```python
from build123d import *

# Parameters (mm, degrees)
SKETCH1_R           = 6
SKETCH1_R_2         = 3.5
BOSS_EXTRUDE1_DEPTH = 2
SKETCH2_R           = 4.5
BOSS_EXTRUDE2_DEPTH = 3
SKETCH3_R           = 2.5
CUT_EXTRUDE1_DEPTH  = 35.398401126
CUT_EXTRUDE2_DEPTH  = 35.398401126


with BuildPart() as part:
    # Sketch1 → Boss-Extrude1 (new body)
    with BuildSketch(Plane.XY):
        Circle(SKETCH1_R)
        with Locations((30, 0)):
            Circle(SKETCH1_R_2)
        Polygon((30, 3.5), (0, 6), (0, -6), (30, -3.5), align=None)
    extrude(amount=BOSS_EXTRUDE1_DEPTH)

    # Sketch2 → Boss-Extrude2 (add)
    with BuildSketch(Plane.XY.offset(2)):
        Circle(SKETCH2_R)
    extrude(amount=BOSS_EXTRUDE2_DEPTH)

    # Sketch3 → Cut-Extrude1 (cut, through all)
    with BuildSketch(Plane.XY.offset(5)):
        Circle(SKETCH3_R)
    extrude(amount=-CUT_EXTRUDE1_DEPTH, mode=Mode.SUBTRACT)

    # Sketch4 → Cut-Extrude2 (cut, through all)
    with BuildSketch(Plane(origin=(0, 0, 0), x_dir=(-1, 0, 0), z_dir=(0, 0, -1))):
        with BuildLine():
            ThreePointArc((-29, 0), (-29.292893219, 0.707106781), (-30, 1))
            Line((-30, 1), (-30, -1))
            ThreePointArc((-30, -1), (-29.292893219, -0.707106781), (-29, 0))
        make_face()
        with BuildLine():
            Line((-30, -1), (-30, 1))
            ThreePointArc((-30, 1), (-31, 0), (-30, -1))
        make_face()
    extrude(amount=-CUT_EXTRUDE2_DEPTH, mode=Mode.SUBTRACT)


solid = part.part
```
Read the model definition and answer for the solid it produces. Units are mm, in the model's axes. Coordinates: 2 decimals unless noted, no trailing zeros. Order: outer loops, then holes, each group sorted by start corner. A loop starts at its lowest first (then second) coordinate and runs counter-clockwise, first axis right, second up. Notation, with made-up numbers: (87.5, 82.25) - (109.5, 82.25) arc R25 ccw to (109.5, 98.25) - close; hole circle Ø7 at (-20, 22.25). An arc over 180 degrees is marked (long way). Answer as a JSON object with one key per item and string values. Group by question number.
Item 1: Section B-B (z = 1.15) is taken. Give the vertices of the cut face in (x, y), plus the area to 3 significant figures.
Item 2: The mould has two halves that part along X. Classify faces 1 (the face through (-0.59, 4.46, 3.48)), 2 (the face through (13, 0, 2)), 3 (the face through (15.7, 4.69, 0.99)), 4 (the face through (-0.54, -2.44, 2.54)): +X half, -X half, draft (parallel to the pull), parting line (faces both ways), or undercut.
Item 3: Consider probe 1 along Y at (x, z) = (0, 3.3); probe 2 along X at (y, z) = (0.5, 2.9); probe 3 along Y at (x, z) = (-1.5, 4). Determine where each line is inside the solid, lowest interval first. Write a range as from..to.
Item 4: Section A-A (x = 0) is taken. Give the vertices of the cut face in (y, z), plus the area to 3 significant figures.
Item 5: Flat-ended cylindrical pins translate along their axes: P1, Ø6, axis at x = 19.5, y = 1, coming from the +Z side; P2, Ø1, axis at y = -3.5, z = 1.5, coming from the +X side; P3, Ø3, axis at x = 0, y = 0, coming from the +Z side. Find the tip coordinate at first contact, or state that the pin passes through.
Item 6: Section D-D (x = 7.5) is taken. Give the vertices of the cut face in (y, z) (3 decimals), plus the area to 3 significant figures.
Item 7: Section C-C (z = 2.85) is taken. Give the vertices of the cut face in (x, y).
Results are:
{
 "1": {"outline": "(0.99, -5.92) - (30, -3.5) arc R3.5 ccw to (30, 3.5) - (0.99, 5.92) arc R6 ccw (long way) to start; hole circle Ø5 at (0, 0); hole circle Ø2 at (30, 0)", "area": "338 mm^2"},
 "2": {"face 1": "parting line", "face 2": "draft", "face 3": "+X half", "face 4": "undercut"},
 "3": {"probe 1": "y = -4.5..-2.5, 2.5..4.5", "probe 2": "x = -4.47..-2.45, 2.45..4.47", "probe 3": "y = -4.24..-2, 2..4.24"},
 "4": {"outline": "(-6, 0) - (-2.5, 0) - (-2.5, 5) - (-4.5, 5) - (-4.5, 2) - (-6, 2) - close; (2.5, 0) - (6, 0) - (6, 2) - (4.5, 2) - (4.5, 5) - (2.5, 5) - close", "area": "26.0 mm^2"},
 "5": {"P1": "stops at z = 2", "P2": "stops at x = 31.8", "P3": "passes through"},
 "6": {"outline": "(-5.375, 0) - (5.375, 0) - (5.375, 2) - (-5.375, 2) - close", "area": "21.5 mm^2"},
 "7": {"outline": "circle Ø9 at (0, 0); hole circle Ø5 at (0, 0)"}
}
